Source: CAD feature listing. Evaluate the final solid. Frame: model axes, mm. Face numbers are marked on the shaded views. Coordinates: 2 decimals unless noted, no trailing zeros. Write each loop counter-clockwise with the first axis right and the second up, starting at its lowest first coordinate (ties: lowest second). Pieces come first, ordered by that corner, then holes. Notation, with made-up numbers: M 60,85.25 L 82,85.25 A29 ccw 82,121.25 Z; hole C -27,-2 d5. An arc over 180 degrees is marked long. Answer as CSV lines item,"result". Start each with the question number.
1. Section B-B on z = -73. Return the cut outline in (x, y), plus the area to 3 significant figures.
2. Section C-C on y = -7. Return the cut outline in (x, z), plus the area to 3 significant figures.
3. Contact query for flat-ended pins moving along their axis: pin 1 Ø4 at (x, z) = (0, -104) entering from -Y; pin 2 Ø2 at (x, y) = (0, -5) entering from -Z; pin 3 Ø2 at (x, y) = (-0.5, 2.5) entering from -Z; pin 4 Ø2 at (x, z) = (2, -93.5) entering from -Y. Output: stop coordinate, or through.
4. Line query: probe 1 along Z at (x, y) = (0, 1.4); probe 2 along X at (y, z) = (1.4, -104); probe 3 along Z at (x, y) = (0, 3.6). Output: solid intervals per line, ascending. Write a range as [from, to].
5. Section A-A on x = 0. Return the cut outline in (y, z), plus the area to 4 significant figures.
6. Mould query, pull axis Z, two halves, no side actions, for the marked faces 1 and 2. Classes: pulls with the +Z half, pulls with the -Z half, needs draft (parallel to the pull), parting line crosses it, or undercut.
Autodesk Inventor part; units mm, degrees
ref_plane "YZ Plane" through (0, 0, 0) normal (1, 0, 0) x (0, 1, 0)
ref_plane "XZ Plane" through (0, 0, 0) normal (0, 1, 0) x (-1, 0, 0)
ref_plane "XY Plane" through (0, 0, 0) normal (0, 0, 1) x (1, 0, 0)
sketch "草圖1" plane through (0, 0, 0) normal (0, 1, 0) x (-1, 0, 0)
  circle A0 centre (0, 0) radius 1.8
  line L0 (0, 0) -> (0, -104) construction
  circle A1 centre (0, -104) radius 1.8
  line L1 (0, -52) -> (-17, -52) construction
  circle A2 centre (0, -104) radius 3.75
  circle A3 centre (0, 0) radius 3.75
  line L2 (-3.75, -104) -> (-3.75, 0)
  line L3 (3.75, -104) -> (3.75, 0)
  line L4 (0, 0) -> (0, -20) construction
  line L5 (0, -104) -> (0, -84) construction
  line L6 (3.75, -84) -> (-3.75, -84)
  line L7 (3.75, -20) -> (-3.75, -20)
  line L8 (0, -20) -> (0, -30) construction
  line L9 (0, -84) -> (0, -74) construction
  line L10 (0, -20) -> (0, -10) construction
  line L11 (0, -84) -> (0, -94) construction
  line L12 (3.75, -94) -> (-3.75, -94)
  line L13 (3.75, -10) -> (-3.75, -10)
  dimension "d0" = 3.6
  dimension "d1" = 104
  dimension "d2" = 3.6
  dimension "d7" = 17
  dimension "d18" = 7.5
  dimension "d19" = 7.5
  dimension "d25" = 20
  dimension "d26" = 20
  dimension "d29" = 10
extrude "Extrusion5" add sketch "草圖1" along normal blind 5 contours A2 | A2 L2 L12 L3 | L12 L2 L6 L3 | L7 L2 L13 L3 | L13 L2 A3 L3 | A3
fillet "Fillet4" radius 2 2 edges at (0, 5, -20) (0, 5, -84)
extrude "Extrusion7" add sketch "草圖1" against normal blind 3 contours L12 L2 L6 L3 | L7 L2 L13 L3
sketch "Sketch2" plane through (0, -3, 0) normal (0, -1, 0) x (1, 0, 0)
  line L0 (3.75, -104) -> (3.75, 0)
  line L1 (-3.75, -104) -> (-3.75, 0)
  line L2 (-3.75, -20) -> (3.75, -20)
  line L3 (3.75, -10) -> (-3.75, -10)
  line L4 (3.75, -84) -> (-3.75, -84)
  line L5 (-3.75, -94) -> (3.75, -94)
  point P0 (0, 0)
extrude "Extrusion8" add sketch "Sketch2" along normal blind 5
fillet "Fillet5" radius 2 6 edges at (0, -8, -94) (0, -8, -10) (0, 0, -10) (0, -3, -20) (0, -3, -84) (0, 0, -94)
properties part number "防傾桿"
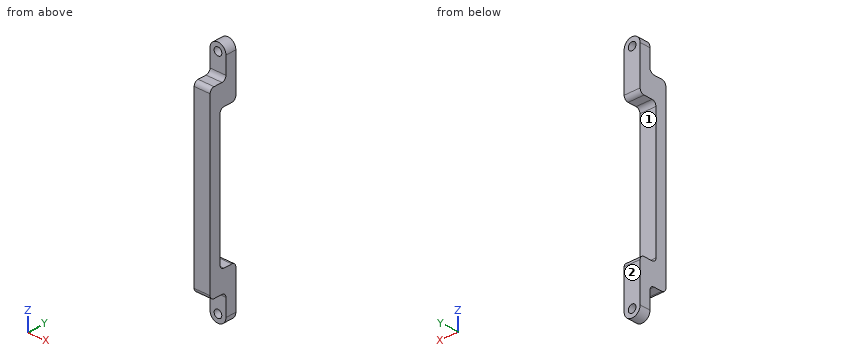
Values:
1,outline,"M -3.75,-8 L 3.75,-8 L 3.75,-3 L -3.75,-3 Z"
1,area,"37.5 mm²"
2,outline,"M -3.75,-93.73 L 3.75,-93.73 L 3.75,-10.27 L -3.75,-10.27 Z"
2,area,"626 mm²"
3,pin 1,"y = 0"
3,pin 2,"z = -94"
3,pin 3,"z = -107.75"
3,pin 4,"y = -7.94"
4,probe 1,"[-107.75, -105.8], [-102.2, -84], [-20, -1.8], [1.8, 3.75]"
4,probe 2,"[-3.75, -1.8], [1.8, 3.75]"
4,probe 3,"[-107.75, -105.8], [-102.2, -84.09], [-19.91, -1.8], [1.8, 3.75]"
5,outline,"M -8,-92 A2 ccw -6,-94 L -2,-94 A2 cw 0,-96 L 0,-102.2 L 5,-102.2 L 5,-86 A2 ccw 3,-84 L -1,-84 A2 cw -3,-82 L -3,-22 A2 cw -1,-20 L 3,-20 A2 ccw 5,-18 L 5,-1.8 L 0,-1.8 L 0,-8 A2 cw -2,-10 L -6,-10 A2 ccw -8,-12 Z; M 0,-107.75 L 5,-107.75 L 5,-105.8 L 0,-105.8 Z; M 0,1.8 L 5,1.8 L 5,3.75 L 0,3.75 Z"
5,area,"681.5 mm²"
6,face 1,"undercut"
6,face 2,"needs draft"
